```python
from build123d import *

# Parameters (mm, degrees)
SKETCH1_R                = 50
BOSS_EXTRUDE1_DEPTH      = 20
BOSS_EXTRUDE2_DEPTH      = 30
BOSS_EXTRUDE2_DEPTH_BACK = 30
CUT_EXTRUDE2_DEPTH       = 30
CHAMFER1_SIZE            = 1.75
CHAMFER1_SIZE2           = 3.031089
SKETCH5_R                = 42
CUT_EXTRUDE3_DEPTH       = 10
FILLET1_R                = 6
FILLET2_R                = 6
FILLET3_R                = 2
FILLET4_R                = 1
SKETCH7_R                = 1
CUT_EXTRUDE5_DEPTH       = 20
CUT_EXTRUDE5_DEPTH_BACK  = 85
SKETCH8_R                = 1
CUT_EXTRUDE6_DEPTH       = 25
CUT_EXTRUDE6_DEPTH_BACK  = 93


with BuildPart() as part:
    # Sketch1 → Boss-Extrude1 (new body)
    with BuildSketch(Plane(origin=(0, 0, 0), x_dir=(1, 0, 0), z_dir=(0, 1, 0))):
        Circle(SKETCH1_R)
    extrude(amount=-BOSS_EXTRUDE1_DEPTH)

    # Sketch3 → Boss-Extrude2 (add, two sides)
    with BuildSketch(Plane(origin=(0, 0, 0), x_dir=(0, 0, -1), z_dir=(1, 0, 0))) as boss_extrude2_sk:
        Polygon((34.980741, -17), (34.980741, -2.160126), (78, -11), (78, -17), align=None)
        Polygon((-78, -11), (-34.980741, -2.160126), (-34.980741, -17), (-78, -17), align=None)
    extrude(amount=BOSS_EXTRUDE2_DEPTH)
    extrude(boss_extrude2_sk.sketch, amount=-BOSS_EXTRUDE2_DEPTH_BACK)

    # Sketch4 → Cut-Extrude2 (cut)
    with BuildSketch(Plane(origin=(0, 0, 0), x_dir=(1, 0, 0), z_dir=(0, 1, 0))):
        with BuildLine():
            Line((22, 78), (-22, 78))
            Line((-22, 78), (-22, 44.899889))
            ThreePointArc((-22, 44.899889), (0, 50), (22, 44.899889))
            Line((22, 44.899889), (22, 78))
        make_face()
        with BuildLine():
            Line((-22, -78), (-22, -44.899889))
            ThreePointArc((-22, -44.899889), (0, -50), (22, -44.899889))
            Line((22, -44.899889), (22, -78))
            Line((22, -78), (-22, -78))
        make_face()
    extrude(amount=-CUT_EXTRUDE2_DEPTH, mode=Mode.SUBTRACT)

    # Chamfer1
    chamfer1_edges = [part.edges().sort_by_distance(p)[0] for p in [
        (0, 0, 50),
    ]]
    chamfer1_side = [part.faces().sort_by_distance(p)[0] for p in [
        (0, -2.700156, 50),
    ]]
    chamfer(chamfer1_edges, length=CHAMFER1_SIZE, length2=CHAMFER1_SIZE2, reference=chamfer1_side[0])

    # Sketch5 → Cut-Extrude3 (cut)
    with BuildSketch(Plane(origin=(0, 0, 0), x_dir=(1, 0, 0), z_dir=(0, 1, 0))):
        Circle(SKETCH5_R)
    extrude(amount=-CUT_EXTRUDE3_DEPTH, mode=Mode.SUBTRACT)

    # Fillet1
    fillet1_edges = [part.edges().sort_by_distance(p)[0] for p in [
        (30, -10.095758, 40),
    ]]
    fillet(fillet1_edges, radius=FILLET1_R)

    # Fillet2
    fillet2_edges = [part.edges().sort_by_distance(p)[0] for p in [
        (-30, -10.095758, 40),
        (30, -10.095758, -40),
        (-30, -10.095758, -40),
    ]]
    fillet(fillet2_edges, radius=FILLET2_R)

    # Fillet3
    fillet3_edges = [part.edges().sort_by_distance(p)[0] for p in [
        (0, -20, 50),
    ]]
    fillet(fillet3_edges, radius=FILLET3_R)

    # Fillet4
    fillet4_edges = [part.edges().sort_by_distance(p)[0] for p in [
        (-30, -14, -78),
        (30, -14, -78),
        (-30, -14, 78),
        (30, -14, 78),
    ]]
    fillet(fillet4_edges, radius=FILLET4_R)

    # Sketch7 → Cut-Extrude5 (cut, two sides)
    with BuildSketch(Plane(origin=(30, 0, 0), x_dir=(0, 0, -1), z_dir=(1, 0, 0))) as cut_extrude5_sk:
        with Locations((-65.06284, -12.670795)):
            Circle(SKETCH7_R)
    extrude(amount=CUT_EXTRUDE5_DEPTH, mode=Mode.SUBTRACT)
    extrude(cut_extrude5_sk.sketch, amount=-CUT_EXTRUDE5_DEPTH_BACK, mode=Mode.SUBTRACT)

    # Sketch8 → Cut-Extrude6 (cut, two sides)
    with BuildSketch(Plane(origin=(30, 0, 0), x_dir=(0, 0, -1), z_dir=(1, 0, 0))) as cut_extrude6_sk:
        with Locations((65.06284, -12.670795)):
            Circle(SKETCH8_R)
    extrude(amount=CUT_EXTRUDE6_DEPTH, mode=Mode.SUBTRACT)
    extrude(cut_extrude6_sk.sketch, amount=-CUT_EXTRUDE6_DEPTH_BACK, mode=Mode.SUBTRACT)


solid = part.part
```
Could you check a few things on this model? Use its own coordinates, in mm. A direction names the side the tool comes from. Coordinates: 2 decimals unless noted, no trailing zeros. Write each loop counter-clockwise with the first axis right and the second up, starting at its lowest first coordinate (ties: lowest second). Pieces come first, ordered by that corner, then holes. Notation, with made-up numbers: M 66,-30.5 L 97,-30.5 A5 ccw 97,-24.5 Z; hole C -10,-18 d1. An arc over 180 degrees is marked long. Answer as CSV lines item,"result". Start each with the question number.
1) I want a section at A-A, the plane z = -54. Please give me the cut outline in (x, y), and give its area (3 significant figures).
2) I want a section at B-B, the plane x = 0. Please give me the cut outline in (y, z), and give its area (3 significant figures).
3) We'd pull the mould along X, two halves only. Please class faces 4 (the conical face through (44.94, -0.085, -14.152)), 5 (the flat face through (-22, -12, -58)), 6 (the flat face through (-1, -10, -1)), 7 (the cylindrical face through (-30.578, -9.822, -40.327)): +X half, -X half, draft (parallel to the pull), parting line (faces both ways), or undercut.
4) Please list where these lines run through material, in increasing order: line 1 (X direction, y = -5.25, z = 45); line 2 (X direction, y = -2.5, z = 0); line 3 (Y direction, x = 3, z = 37). Write a range as from..to.
5) For P1, Ø10, axis at y = -8, z = 57.5, coming from the +X side; P2, Ø4, axis at y = -17.5, z = 34, coming from the -X side; P3, Ø10, axis at x = 12, z = -26, coming from the +Y side, each with a flat end and sliding along its axis, tell me the tip position at first contact or that it passes through.
6) For faces 1 (the flat face through (30, -12, 56)), 2 (the flat face through (-25.873, -6.864, -57.872)), 3 (the flat face through (26, -17, -58)), which set-ups out of +Z, -Z, +X, -X, +Y, -Y let a thin tool reach every point of the face, with its end or its side?
7) I want a section at C-C, the plane z = 0. Please give me the cut outline in (x, y), and give its area (3 significant figures).
Data:
1,outline,"M -30,-17 L -22,-17 L -22,-6.07 L -30,-6.07 Z; M 22,-17 L 30,-17 L 30,-6.07 L 22,-6.07 Z"
1,area,"175 mm^2"
2,outline,"M -20,-48 A2 ccw -18,-50 L -1.75,-50 L 0,-46.97 L 0,-42 L -10,-42 L -10,42 L 0,42 L 0,46.97 L -1.75,50 L -18,50 A2 ccw -20,48 Z"
2,area,"1,150 mm^2"
3,face 4,"parting line"
3,face 5,"undercut"
3,face 6,"undercut"
3,face 7,"-X half"
4,line 1,"x = -30..-22, -21.79..21.79, 22..30"
4,line 2,"x = -50..-42, 42..50"
4,line 3,"y = -20..-10"
5,P1,"stops at x = 30"
5,P2,"stops at x = -38.42"
5,P3,"stops at y = -10"
6,face 1,"+Z, +X, +Y, -Y"
6,face 2,"-Z, -X, +Y"
6,face 3,"-Z, +X, -Y"
7,outline,"M -50,-18 A2 ccw -48,-20 L 48,-20 A2 ccw 50,-18 L 50,-1.75 L 46.97,0 L 42,0 L 42,-10 L -42,-10 L -42,0 L -46.97,0 L -50,-1.75 Z"
7,area,"1,150 mm^2"
